Could you check a few things on this model? Use its own coordinates, in mm. Face numbers are marked on the shaded views. A direction names the side the tool comes from. Give positions to 0.01 mm unless a question says otherwise; leave off trailing zeros. Write each loop counter-clockwise with the first axis right and the second up, starting at its lowest first coordinate (ties: lowest second). Pieces come first, ordered by that corner, then holes. Notation, with made-up numbers: (-16, -4) - (22, -4) arc R15 cw to (22, 22) - close; hole circle Ø11 at (63, -22.5). An arc over 180 degrees is marked (long way). Answer as CSV lines item,"result". Start each with the question number.
Q1. On a 3-axis mill with a long thin cutter (end or side, diameter ignored), from which of +Z, -Z, +X, -X, +Y, -Y can I reach the whole of each face in a straight line? I mean the marked faces 1, 2 and 3. Say none if no direction works.
Q2. Imagine slicing it at B-B on z = 0. List the corners of the cut face in (x, y) for me, and give its area (3 significant figures).
Q3. Imagine slicing it at D-D on y = 5.75. List the corners of the cut face in (x, z) for me, and give its area (3 significant figures).
Q4. Will these pins go through, and if not, where does the flat tip stop? pin 1 Ø2 at (y, z) = (6, -2.5) entering from -X; pin 2 Ø2.5 at (x, z) = (-4.5, -1) entering from +Y; pin 3 Ø0.6 at (y, z) = (6, 1) entering from +X.
Q5. If I drill on line 1 along Z through (x, y) = (0, 5.25); line 2 along X through (y, z) = (2, 0.5); line 3 along Z through (x, y) = (-1.75, 2.75), over which ranges is the centre line in solid material (lowest first)?
Q6. Imagine slicing it at C-C on z = 3. List the corners of the cut face in (x, y) for me.
Q7. Imagine slicing it at A-A on x = 0. List the corners of the cut face in (y, z) for me.
```python
from build123d import *

# Parameters (mm, degrees)
BOSS_EXTRUDE1_DEPTH = 7.5
M6_TAPPED_HOLE1_D   = 5
FILLET1_R           = 2


with BuildPart() as part:
    # Sketch2 → Boss-Extrude1 (new, symmetric)
    with BuildSketch(Plane.XY):
        Polygon((-6, 5.196152423), (-3, 0), (3, 0), (6, 5.196152423), (3, 5.196152423), (3, 7.196152423), (-3, 7.196152423), (-3, 5.196152423), align=None)
    extrude(amount=BOSS_EXTRUDE1_DEPTH, both=True)

    # M6 Tapped Hole1 (through all)
    with Locations(Plane(origin=(0, 7.196152423, 0), x_dir=(1, 0, 0), z_dir=(0, 1, 0))):
        with Locations((0, 0)):
            Hole(M6_TAPPED_HOLE1_D / 2)

    # Fillet1
    # the kernel refuses this fillet: 2 mm, written as the material it takes off along each edge
    with BuildSketch(Plane(origin=(3, 0, -10.386751346), x_dir=(-1, 0, 0), z_dir=(0, 0, 1)), Plane(origin=(-3, 0, -10.386751346), x_dir=(-0.5000000000000046, 0.866025403784436, 0), z_dir=(0, 0, 1))) as fillet1_piece_1:
        with BuildLine():
            CenterArc((FILLET1_R * 0.57735026919, -FILLET1_R), FILLET1_R, 90, 60)
            Line((-FILLET1_R * 0.288675134595, -FILLET1_R * 0.5), (0, 0))
            Line((0, 0), (FILLET1_R * 0.57735026919, 0))
        make_face()
    extrude(amount=20.773502692, mode=Mode.SUBTRACT)


solid = part.part
```
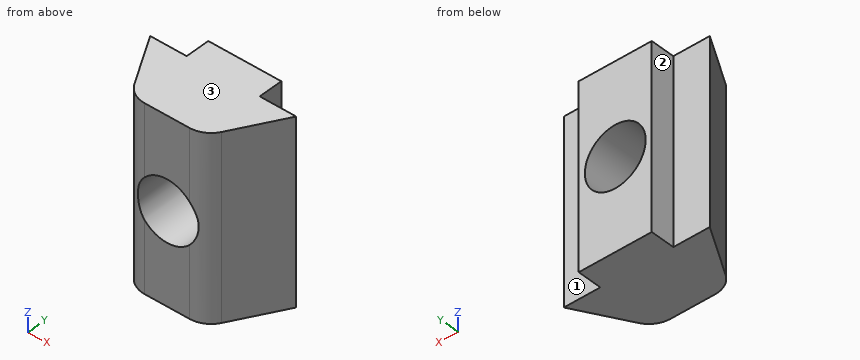
Conclusion:
1,face 1,"+Z, -Z, +X, +Y"
1,face 2,"+Z, -Z, -X, +Y"
1,face 3,"+Z, +X, -X, +Y, -Y"
2,outline,"(-6, 5.2) - (-3.58, 1) arc R2 ccw to (-2.5, 0.11) - (-2.5, 7.2) - (-3, 7.2) - (-3, 5.2) - close; (2.5, 0.11) arc R2 ccw to (3.58, 1) - (6, 5.2) - (3, 5.2) - (3, 7.2) - (2.5, 7.2) - close"
2,area,"22.4 mm^2"
3,outline,"(-3, -7.5) - (3, -7.5) - (3, 7.5) - (-3, 7.5) - close; hole circle Ø5 at (0, 0)"
3,area,"70.4 mm^2"
4,pin 1,"x = -6"
4,pin 2,"y = 5.2"
4,pin 3,"x = 3"
5,line 1,"-7.5 to -2.5, 2.5 to 7.5"
5,line 2,"-4.15 to -2.45, 2.45 to 4.15"
5,line 3,"-7.5 to -1.79, 1.79 to 7.5"
6,outline,"(-6, 5.2) - (-3.58, 1) arc R2 ccw to (-1.85, 0) - (1.85, 0) arc R2 ccw to (3.58, 1) - (6, 5.2) - (3, 5.2) - (3, 7.2) - (-3, 7.2) - (-3, 5.2) - close"
7,outline,"(0, -7.5) - (7.2, -7.5) - (7.2, -2.5) - (0, -2.5) - close; (0, 2.5) - (7.2, 2.5) - (7.2, 7.5) - (0, 7.5) - close"
